Input: dimensioned drawing with shaded views. Units: mm. Origin: part minimum x, y, z. Coordinates: 2 decimals unless noted, no trailing zeros. Use CSV: the item, a comma, the result in double quotes. Start each with the question number.
1. Section query A-A on z = 71. State how many separate pieces and enclosed holes the cut face has, and give its area (3 significant figures).
2. First-contact query: P1, Ø1, axis at x = 326, z = 41, coming from the +Y side; P2, Ø1, axis at y = 107, z = 44, coming from the -X side. Flat tips, straight axial feed; report the tip coordinate or a pass-through.
3. Material intervals for line 1 (Y direction, x = 1158, z = 58); line 2 (X direction, y = 487, z = 83.5), sorted ascending.
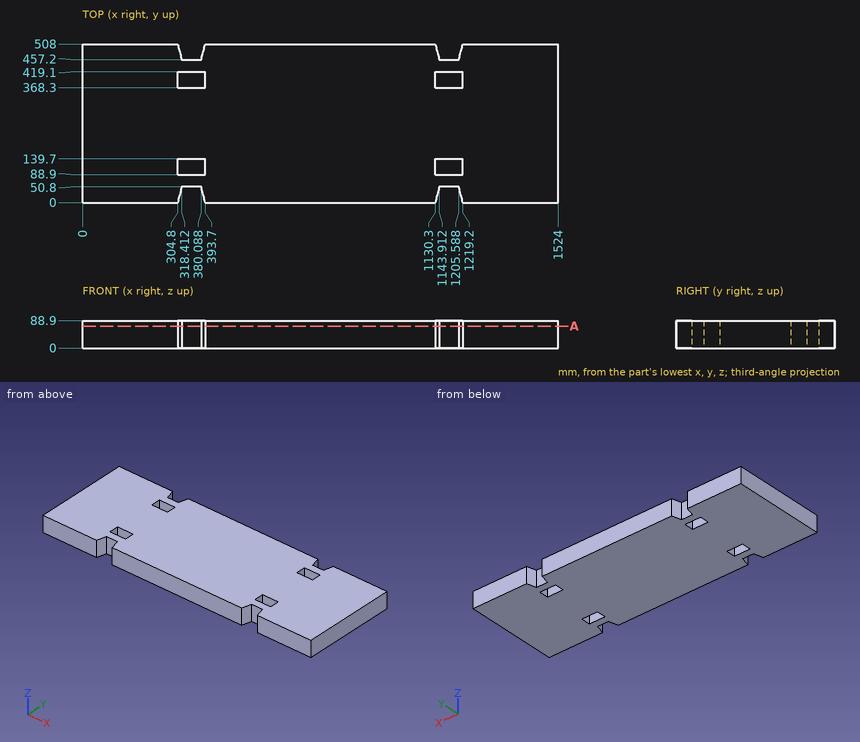
Results list:
1,separate pieces,"1"
1,enclosed holes,"4"
1,area,"741,000 mm²"
2,P1,"stops at y = 457.2"
2,P2,"stops at x = 0"
3,line 1,"y = 50.8 to 88.9, 139.7 to 368.3, 419.1 to 457.2"
3,line 2,"x = 0 to 310.43, 388.07 to 1135.93, 1213.57 to 1524"
